Input: part model. Units: mm. Frame: model coordinates. Face numbers are marked on the shaded views. A direction names the side the tool comes from. Give positions to 0.01 mm unless a question says otherwise; leave off trailing zeros. Write each loop counter-clockwise with the first axis right and the second up, starting at its lowest first coordinate (ties: lowest second). Pieces come first, ordered by that corner, then holes.
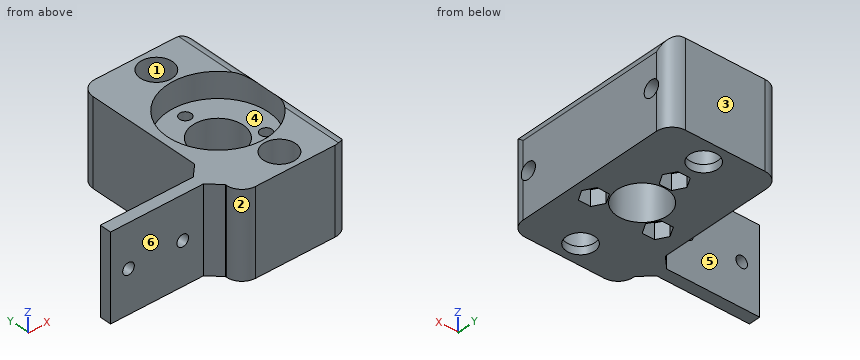
```python
from build123d import *

# Parameters (mm, degrees)
SKETCH1_W           = 28.5
SKETCH1_H           = 47
SKETCH1_R           = 3.65
SKETCH1_R_2         = 13
BOSS_EXTRUDE1_DEPTH = 2
SKETCH1_3_W         = 28.5
SKETCH1_3_H         = 47
SKETCH1_3_R         = 4.15
SKETCH1_3_R_2       = 13
BOSS_EXTRUDE2_DEPTH = 22
SKETCH2_W           = 22
SKETCH2_H           = 3
BOSS_EXTRUDE3_DEPTH = 27
SKETCH1_4_R         = 13
SKETCH1_4_R_2       = 6.5
BOSS_EXTRUDE4_DEPTH = 15.5
SKETCH3_R           = 1.5
CUT_EXTRUDE1_DEPTH  = 51.561843321
CUT_EXTRUDE3_REACH  = 66.16
SKETCH5_R           = 2.1
CUT_EXTRUDE4_REACH  = 71.16
CUT_EXTRUDE4_START  = -5
SKETCH5_3_R         = 2.1
CUT_EXTRUDE5_REACH  = 61.957
SKETCH6_R           = 1.5
CHAMFER1_SIZE       = 3
FILLET1_R           = 4
FILLET2_R           = 3
CUT_EXTRUDE6_DEPTH  = 4


with BuildPart() as part:
    # Sketch1 → Boss-Extrude1 (new body)
    with BuildSketch(Plane.XY):
        with Locations((-0.75, 0)):
            Rectangle(SKETCH1_W, SKETCH1_H)
        with Locations((0, 18)):
            Circle(SKETCH1_R, mode=Mode.SUBTRACT)
        with Locations((0, -18)):
            Circle(SKETCH1_R, mode=Mode.SUBTRACT)
        Circle(SKETCH1_R_2, mode=Mode.SUBTRACT)
    extrude(amount=BOSS_EXTRUDE1_DEPTH)

    # Sketch1<3> → Boss-Extrude2 (add)
    with BuildSketch(Plane.XY):
        with Locations((-0.75, 0)):
            Rectangle(SKETCH1_3_W, SKETCH1_3_H)
        with Locations((0, 18)):
            Circle(SKETCH1_3_R, mode=Mode.SUBTRACT)
        with Locations((0, -18)):
            Circle(SKETCH1_3_R, mode=Mode.SUBTRACT)
        Circle(SKETCH1_3_R_2, mode=Mode.SUBTRACT)
    extrude(amount=BOSS_EXTRUDE2_DEPTH)

    # Sketch2 → Boss-Extrude3 (add)
    with BuildSketch(Plane.ZY.offset(15)):
        with Locations((11, -14.7)):
            Rectangle(SKETCH2_W, SKETCH2_H)
    extrude(amount=BOSS_EXTRUDE3_DEPTH)

    # Sketch1<4> → Boss-Extrude4 (add)
    with BuildSketch(Plane.XY):
        Circle(SKETCH1_4_R)
        Circle(SKETCH1_4_R_2, mode=Mode.SUBTRACT)
    extrude(amount=BOSS_EXTRUDE4_DEPTH)

    # Sketch3 → Cut-Extrude1 (cut, through all)
    with BuildSketch(Plane.XY.offset(15.5)):
        with Locations((0, 9.525)):
            Circle(SKETCH3_R)
        with Locations((8.248891971, -4.7625)):
            Circle(SKETCH3_R)
        with Locations((-8.248891971, -4.7625)):
            Circle(SKETCH3_R)
    extrude(amount=-CUT_EXTRUDE1_DEPTH, mode=Mode.SUBTRACT)

    # Sketch5 → Cut-Extrude3 (cut, up to next)
    with BuildSketch(Plane(origin=(13.5, 0, 0), x_dir=(0, 0, -1), z_dir=(1, 0, 0)), mode=Mode.PRIVATE) as cut_extrude3_sk1:
        with Locations((-11, 18)):
            Circle(SKETCH5_R)
    cut_extrude3_tool1 = extrude(cut_extrude3_sk1.sketch, amount=-CUT_EXTRUDE3_REACH, mode=Mode.PRIVATE) & part.part
    # Sketch5 → Cut-Extrude3 (cut, up to next)
    with BuildSketch(Plane(origin=(13.5, 0, 0), x_dir=(0, 0, -1), z_dir=(1, 0, 0)), mode=Mode.PRIVATE) as cut_extrude3_sk2:
        with Locations((-11, -18)):
            Circle(SKETCH5_R)
    cut_extrude3_tool2 = extrude(cut_extrude3_sk2.sketch, amount=-CUT_EXTRUDE3_REACH, mode=Mode.PRIVATE) & part.part
    add(cut_extrude3_tool1.solids().sort_by_distance((13.5, 18, 11))[0], mode=Mode.SUBTRACT)
    add(cut_extrude3_tool2.solids().sort_by_distance((13.5, -18, 11))[0], mode=Mode.SUBTRACT)

    # Sketch5<3> → Cut-Extrude4 (cut, up to next)
    with BuildSketch(Plane(origin=(13.5, 0, 0), x_dir=(0, 0, -1), z_dir=(1, 0, 0)).offset(CUT_EXTRUDE4_START), mode=Mode.PRIVATE) as cut_extrude4_sk1:
        Polygon((-6.958548116, 18), (-8.979274058, 21.5), (-13.020725942, 21.5), (-15.041451884, 18), (-13.020725942, 14.5), (-8.979274058, 14.5), align=None)
        with Locations((-11, 18)):
            Circle(SKETCH5_3_R, mode=Mode.SUBTRACT)
    cut_extrude4_tool1 = extrude(cut_extrude4_sk1.sketch, amount=-CUT_EXTRUDE4_REACH, mode=Mode.PRIVATE) & part.part
    # Sketch5<3> → Cut-Extrude4 (cut, up to next)
    with BuildSketch(Plane(origin=(13.5, 0, 0), x_dir=(0, 0, -1), z_dir=(1, 0, 0)).offset(CUT_EXTRUDE4_START), mode=Mode.PRIVATE) as cut_extrude4_sk2:
        Polygon((-6.958548116, -18), (-8.979274058, -14.5), (-13.020725942, -14.5), (-15.041451884, -18), (-13.020725942, -21.5), (-8.979274058, -21.5), align=None)
        with Locations((-11, -18)):
            Circle(SKETCH5_3_R, mode=Mode.SUBTRACT)
    cut_extrude4_tool2 = extrude(cut_extrude4_sk2.sketch, amount=-CUT_EXTRUDE4_REACH, mode=Mode.PRIVATE) & part.part
    add(cut_extrude4_tool1.solids().sort_by_distance((8.5, 19.696537, 8.061512))[0], mode=Mode.SUBTRACT)
    add(cut_extrude4_tool2.solids().sort_by_distance((8.5, -16.303463, 8.061512))[0], mode=Mode.SUBTRACT)

    # Sketch6 → Cut-Extrude5 (cut, up to next)
    with BuildSketch(Plane(origin=(0, -13.2, 0), x_dir=(1, 0, 0), z_dir=(0, 1, 0)), mode=Mode.PRIVATE) as cut_extrude5_sk1:
        with Locations(Location((-37.367, -11, 0), (0, 0, 270))):
            Circle(SKETCH6_R)
    cut_extrude5_tool1 = extrude(cut_extrude5_sk1.sketch, amount=-CUT_EXTRUDE5_REACH, mode=Mode.PRIVATE) & part.part
    # Sketch6 → Cut-Extrude5 (cut, up to next)
    with BuildSketch(Plane(origin=(0, -13.2, 0), x_dir=(1, 0, 0), z_dir=(0, 1, 0)), mode=Mode.PRIVATE) as cut_extrude5_sk2:
        with Locations(Location((-23.367, -11, 0), (0, 0, 270))):
            Circle(SKETCH6_R)
    cut_extrude5_tool2 = extrude(cut_extrude5_sk2.sketch, amount=-CUT_EXTRUDE5_REACH, mode=Mode.PRIVATE) & part.part
    add(cut_extrude5_tool1.solids().sort_by_distance((-37.367, -13.2, 11))[0], mode=Mode.SUBTRACT)
    add(cut_extrude5_tool2.solids().sort_by_distance((-23.367, -13.2, 11))[0], mode=Mode.SUBTRACT)

    # Chamfer1
    chamfer1_edges = [part.edges().sort_by_distance(p)[0] for p in [
        (-15, -16.2, 11),
        (-15, -13.2, 11),
    ]]
    chamfer(chamfer1_edges, length=CHAMFER1_SIZE)

    # Fillet1
    # the kernel refuses this fillet: 4 mm, written as the material it takes off along each edge
    with BuildSketch(Plane(origin=(-15, -23.5, 32), x_dir=(0, 1, 0), z_dir=(0, 0, -1)), Plane(origin=(-15, 23.5, 32), x_dir=(1, 0, 0), z_dir=(0, 0, -1))) as fillet1_piece_1:
        with BuildLine():
            CenterArc((FILLET1_R, FILLET1_R), FILLET1_R, 180, 90)
            Line((0, FILLET1_R), (0, 0))
            Line((0, 0), (FILLET1_R, 0))
        make_face()
    extrude(amount=42, mode=Mode.SUBTRACT)
    with BuildSketch(Plane(origin=(13.5, 23.5, -10), x_dir=(0, -1, 0), z_dir=(0, 0, 1)), Plane(origin=(13.5, -23.5, -10), x_dir=(-1, 0, 0), z_dir=(0, 0, 1))) as fillet1_piece_2:
        with BuildLine():
            CenterArc((FILLET1_R, -FILLET1_R), FILLET1_R, 90, 90)
            Line((0, -FILLET1_R), (0, 0))
            Line((0, 0), (FILLET1_R, 0))
        make_face()
    extrude(amount=42, mode=Mode.SUBTRACT)

    # Fillet2
    # the kernel refuses this fillet: 3 mm, written as the material it takes off along each edge
    with BuildSketch(Plane(origin=(13.5, -27, 22), x_dir=(-1, 0, 0), z_dir=(0, 1, 0))) as fillet2_piece_1:
        with BuildLine():
            CenterArc((FILLET2_R, -FILLET2_R), FILLET2_R, 90, 90)
            Line((0, -FILLET2_R), (0, 0))
            Line((0, 0), (FILLET2_R, 0))
        make_face()
    extrude(amount=54, mode=Mode.SUBTRACT)

    # Sketch7 → Cut-Extrude6 (cut)
    with BuildSketch(Plane(origin=(0, 0, 0), x_dir=(-1, 0, 0), z_dir=(0, 0, -1))):
        Polygon((1.58771324, 6.775), (3.175426481, 9.525), (1.58771324, 12.275), (-1.58771324, 12.275), (-3.175426481, 9.525), (-1.58771324, 6.775), align=None)
        Polygon((11.424318452, -4.7625), (9.836605211, -2.0125), (6.661178731, -2.0125), (5.073465491, -4.7625), (6.661178731, -7.5125), (9.836605211, -7.5125), align=None)
        Polygon((-9.836605211, -7.5125), (-6.661178731, -7.5125), (-5.073465491, -4.7625), (-6.661178731, -2.0125), (-9.836605211, -2.0125), (-11.424318452, -4.7625), align=None)
    extrude(amount=-CUT_EXTRUDE6_DEPTH, mode=Mode.SUBTRACT)


solid = part.part
```
Item 1: Section D-D (y = -4). Return loops of the section in (x, z), and give its area (3 significant figures).
Item 2: Mould query, pull axis X, two halves, no side actions, for the marked faces 1, 2 and 3. Classes: +X half, -X half, draft (parallel to the pull), parting line (faces both ways), or undercut.
Item 3: Section A-A (x = 0). Give the number of separate pieces and of enclosed holes in the cut face, and give its area (3 significant figures).
Item 4: Section B-B (y = 3.5). Return loops of the section in (x, z).
Item 5: Ray query, line 1 (Y direction, x = 0, z = 1.15) (3 decimals); line 2 (Y direction, x = 0, z = 19.75); line 3 (Y direction, x = 5, z = 13). Return the intervals inside material, ascending.
Item 6: Set-up query: the marked faces 4, 5 and 6. Return all of +Z, -Z, +X, -X, +Y, -Y with unobstructed straight access to the full face (end or side cutting, diameter ignored); none if empty.
Item 7: Pin query (flat end, axial travel): pin 1 (4 mm diameter, centred on x = -31, z = 10.5, fed in from -Y); pin 2 (12 mm diameter, centred on x = -34, z = 11.5, fed in from +Y); pin 3 (3.5 mm diameter, centred on y = 18, z = 11, fed in from +X). Return the tip coordinate at first contact, or that it passes through.
Solved:
1. outline: (-15, 0) - (-10.98, 0) - (-10.98, 4) - (-9.54, 4) - (-9.54, 15.5) - (-12.37, 15.5) - (-12.37, 22) - (-15, 22) - close; (-6.96, 4) - (-5.51, 4) - (-5.51, 0) - (-5.12, 0) - (-5.12, 15.5) - (-6.96, 15.5) - close; (5.12, 0) - (5.51, 0) - (5.51, 4) - (6.96, 4) - (6.96, 15.5) - (5.12, 15.5) - close; (9.54, 4) - (10.98, 4) - (10.98, 0) - (13.5, 0) - (13.5, 19) arc R3 ccw to (12.37, 21.35) - (12.37, 15.5) - (9.54, 15.5) - close
1. area: 203 mm2
2. face 1: undercut
2. face 2: -X half
2. face 3: draft
3. separate pieces: 5
3. enclosed holes: 0
3. area: 246 mm2
4. outline: (-15, 0) - (-5.48, 0) - (-5.48, 15.5) - (-12.52, 15.5) - (-12.52, 22) - (-15, 22) - close; (5.48, 0) - (13.5, 0) - (13.5, 19) arc R3 ccw to (12.52, 21.22) - (12.52, 15.5) - (5.48, 15.5) - close
5. line 1: y = -23.5 to -21.65, -14.35 to -6.5, 6.5 to 6.775, 12.275 to 14.35, 21.65 to 23.5
5. line 2: y = -23.5 to -22.15, -13.85 to -13, 13 to 13.85, 22.15 to 23.5
5. line 3: y = -23.5 to -21.5, -14.5 to -4.15, 4.15 to 14.5, 21.5 to 23.5
6. face 4: +Z
6. face 5: +Z, -Z, -X, +Y
6. face 6: +Z, -Z, -X, -Y
7. pin 1: stops at y = -16.2
7. pin 2: stops at y = -13.2
7. pin 3: stops at x = -3.76
